```python
from build123d import *

# Parameters (mm, degrees)
F1_DEPTH = 9.525
F3_DEPTH = 9.526
F4_R     = 10.16
F5_R     = 3.175
F6_DEPTH = 12.7
F7_R     = 3.175
F8_DEPTH = 12.7


with BuildPart() as f1:
    # F0 (on Front) → F1 (new body)
    with BuildSketch(Plane.XZ):
        Polygon((-50.537063, 64.119838), (-75.937063, 64.119838), (-75.937063, -62.880162), (19.312937, -62.880162), (19.312937, -37.480162), align=None)
    extrude(amount=F1_DEPTH)

    # F2 (on face) → F3 (cut, through all)
    with BuildSketch(Plane.XZ.offset(9.525)):
        Polygon((0, -43.830162), (-56.887063, 38.914657), (-56.887063, -43.830162), align=None)
    extrude(amount=-F3_DEPTH, mode=Mode.SUBTRACT)

    # F4
    f4_edges = [f1.edges().sort_by_distance(p)[0] for p in [
        (-56.887063, -4.7625, -43.830162),
        (0, -4.7625, -43.830162),
        (-56.887063, -4.7625, 38.914657),
    ]]
    fillet(f4_edges, radius=F4_R)

    # F5 (on face) → F6 (cut)
    with BuildSketch(Plane(origin=(0, 0, -62.880162), x_dir=(1, 0, 0), z_dir=(0, 0, -1))):
        with Locations((-56.887063, 4.7752)):
            Circle(F5_R)
        with Locations((-28.312063, 4.7498)):
            Circle(F5_R)
        with Locations((0.262937, 4.7752)):
            Circle(F5_R)
    extrude(amount=-F6_DEPTH, mode=Mode.SUBTRACT)

    # F7 (on face) → F8 (cut)
    with BuildSketch(Plane(origin=(-75.937063, 0, 0), x_dir=(0, -1, 0), z_dir=(-1, 0, 0))):
        with Locations((4.7498, 45.069838)):
            Circle(F7_R)
        with Locations((4.7498, 0.619838)):
            Circle(F7_R)
        with Locations((4.7498, -43.830162)):
            Circle(F7_R)
    extrude(amount=-F8_DEPTH, mode=Mode.SUBTRACT)


solid = f1.part
```
Verification items for the finished model (mm, model axes). A direction names the side the tool comes from. Round coordinates to 2 decimals unless told otherwise and drop trailing zeros. Order: outer loops, then holes, each group sorted by start corner. A loop starts at its lowest first (then second) coordinate and runs counter-clockwise, first axis right, second up. Notation, with made-up numbers: (15, 54.5) - (35, 54.5) arc R29 ccw to (35, 87.5) - close; hole circle Ø11 at (63, 55). An arc over 180 degrees is marked (long way). Use CSV: the item, a comma, the result in double quotes. Start each with the question number.
1) Section check B-B, the plane x = -33.5. Record the cut outline in (y, z) (3 decimals), plus the area to 3 significant figures.
2) Go/stop test with flat-tipped pins: P1, Ø5, axis at x = 0.26, y = -4.78, coming from the +Z side; P2, Ø3, axis at x = -2, y = -1, coming from the +Z side; P3, Ø3, axis at x = -57, y = -4, coming from the -Z side. Record where each tip stops, or that it passes through.
3) Mould release check, pull along Z, two halves, no side actions. Record for faces 6 (the flat face through (-28, -5, -50.18)), 7 (the cylindrical face through (-25.38, -3.53, -56.62)), 8 (the cylindrical face through (-53.99, -4.696, -40.775)): +Z half, -Z half, draft (parallel to the pull), parting line (faces both ways), or undercut.
4) Section check D-D, the plane x = -68. Record the cut outline in (y, z) (3 decimals).
5) Access from +Z, -Z, +X, -X, +Y, -Y to the whole of each face (thin tool, end or side, straight path). Record for faces 1 (the cylindrical face through (-0.425, -1.676, -56.619)), 2 (the flat face through (-56.887, -5, -13)), 3 (the flat face through (-29, -9, -62.88)), 4 (the flat face through (-63.237, -5, 1)), 5 (the flat face through (-75.937, -1.5, 1.5)).
6) Thickness scan on L1, parallel to X at y = -7.5, z = -55.5; L2, parallel to X at y = -7.25, z = -40; L3, parallel to Z at x = -53, y = -5.75. Record the ranges inside material, lowest first.
7) Section check C-C, the plane z = -51.5. Record the cut outline in (x, y) (3 decimals), plus the area to 3 significant figures.
8) Section check A-A, the plane z = -16.5. Record the cut outline in (x, y) (3 decimals).
Answers:
1,outline,"(-9.525, -62.88) - (0, -62.88) - (0, -43.83) - (-9.525, -43.83) - close; (-9.525, 4.897) - (0, 4.897) - (0, 39.339) - (-9.525, 39.339) - close"
1,area,"510 mm²"
2,P1,"stops at z = -6.13"
2,P2,"stops at z = -4.3"
2,P3,"stops at z = -50.18"
3,face 6,"-Z half"
3,face 7,"draft"
3,face 8,"undercut"
4,outline,"(-9.525, -62.88) - (0, -62.88) - (0, 64.12) - (-9.525, 64.12) - close; hole circle Ø6.35 at (-4.75, -43.83); hole circle Ø6.35 at (-4.75, 0.62); hole circle Ø6.35 at (-4.75, 45.07)"
5,face 1,"-Z"
5,face 2,"+Y, -Y"
5,face 3,"-Z, +X, -X, +Y, -Y"
5,face 4,"-X"
5,face 5,"+Z, -Z, -X, +Y, -Y"
6,L1,"x = -75.94 to -58.52, -55.26 to -29.9, -26.73 to -1.37, 1.89 to 19.31"
6,L2,"x = -75.94 to -54.67, -11.37 to 19.31"
6,L3,"z = -62.88 to -41.66, 14.19 to 64.12"
7,outline,"(-75.937, -9.525) - (19.313, -9.525) - (19.313, 0) - (-75.937, 0) - close; hole circle Ø6.35 at (-56.887, -4.775); hole circle Ø6.35 at (-28.312, -4.75); hole circle Ø6.35 at (0.263, -4.775)"
7,area,"812 mm²"
8,outline,"(-75.937, -9.525) - (-56.887, -9.525) - (-56.887, 0) - (-75.937, 0) - close; (-18.789, -9.525) - (4.889, -9.525) - (4.889, 0) - (-18.789, 0) - close"
